from build123d import *

# Parameters (mm, degrees)
F1_DEPTH = 8
F2_R     = 3.99999
F3_R     = 1
F4_DEPTH = 60
F6_R     = 3.99999
F5_R     = 3.5
F7_DEPTH = 2
F8_R     = 0.75
F9_DEPTH = 12


# Not quite as in the source:
# - a fillet or chamfer is up to 0.001 mm smaller than in the source, because OpenCascade refuses the exact size


with BuildPart() as f1:
    # F0 (on Top) → F1 (new body)
    with BuildSketch(Plane.XY):
        Polygon((-9.9077894302, -1.920078908), (-9.9077894302, -12.520078908), (8.0922105698, -12.520078908), (8.0922105698, -0.520078908), (28.0922105698, -0.520078908), (28.0922105698, 10.079921092), (14.0922105698, 10.079921092), (14.0922105698, 22.579921092), (28.0922105698, 22.579921092), (28.0922105698, 33.179921092), (-9.9077894302, 33.179921092), (-9.9077894302, 22.579921092), (0.0922105698, 22.579921092), (0.0922105698, -1.920078908), align=None)
    extrude(amount=F1_DEPTH)

    # F2 (radius 4 in the source; OpenCascade refuses exactly that, so slightly less here)
    f2_edges = [f1.edges().sort_by_distance(p)[0] for p in [
        (-9.907789, -7.220079, 8),
        (-9.907789, -7.220079, 0),
        (8.092211, -6.520079, 8),
        (8.092211, -6.520079, 0),
        (28.092211, 4.779921, 8),
        (28.092211, 4.779921, 0),
        (28.092211, 27.879921, 8),
        (28.092211, 27.879921, 0),
        (-9.907789, 27.879921, 8),
        (-9.907789, 27.879921, 0),
    ]]
    fillet(f2_edges, radius=F2_R)

    # F3 (on face) → F4 (cut)
    with BuildSketch(Plane(origin=(0, 33.179921092, 0), x_dir=(-1, 0, 0), z_dir=(0, 1, 0))):
        with Locations((-24.0922105698, 4)):
            Circle(F3_R)
        with Locations((5.9077894302, 4)):
            Circle(F3_R)
    extrude(amount=-F4_DEPTH, mode=Mode.SUBTRACT)

    # F6 (radius 4 in the source; OpenCascade refuses exactly that, so slightly less here)
    f6_edges = [f1.edges().sort_by_distance(p)[0] for p in [
        (0.092211, 10.329921, 8),
        (0.092211, 10.329921, 0),
        (14.092211, 16.329921, 8),
        (14.092211, 16.329921, 0),
    ]]
    fillet(f6_edges, radius=F6_R)

    # F5 (on face) → F7 (join)
    with BuildSketch(Plane.XZ.offset(0.520078908)):
        with Locations((17.0922105698, 4)):
            Circle(F5_R)
    extrude(amount=F7_DEPTH)

    # F8 (on face) → F9 (cut)
    with BuildSketch(Plane.XZ.offset(2.520078908)):
        with Locations((17.0922105698, 4)):
            Circle(F8_R)
    extrude(amount=-F9_DEPTH, mode=Mode.SUBTRACT)


solid = f1.part
Work out the finished part from the listing and answer in its coordinate system (mm). A direction names the side the tool comes from. Coordinates: 2 decimals unless noted, no trailing zeros. Write each loop counter-clockwise with the first axis right and the second up, starting at its lowest first coordinate (ties: lowest second). Pieces come first, ordered by that corner, then holes. Notation, with made-up numbers: M 88,61 L 124,61 A29 cw 124,83 Z; hole C -13.5,80 d3. An arc over 180 degrees is marked long. Use one line per item in the form item = value. Start each with the question number.
1. The part is cut by section A-A (y = 30.5). Give the number of separate pieces and of enclosed holes in the cut face, plus the area to 3 significant figures.
2. Each of these flat-tipped pins is pushed along its axis until it touches: P1, Ø4, axis at y = 19.5, z = 5, coming from the -X side; P2, Ø1.2, axis at x = 17, z = 4, coming from the -Y side; P3, Ø4, axis at x = 14.5, z = 2.5, coming from the -Y side. Where does it stop, or does it pass through?
3. The mould has two halves that part along Y. Classify faces 4 (the face through (26.95, 4.85, 6.8)), 5 (the face through (1.295, 10.158, 1.141)), 6 (the face through (15.9, -0.52, 7.5)): released by +Y, released by -Y, zero draft, split by the parting line, or undercut.
4. A tool of negligible diameter and unlimited length cuts with its end or side. For faces 1 (the face through (12.89, 16.42, 6.86)), 2 (the face through (6.95, -6.44, 1.2)), 3 (the face through (1.295, 10.158, 6.859)), from which of +Z, -Z, +X, -X, +Y, -Y can it reach the whole face along a straight path? Write none if from no direction.
5. Straight lines are drawn through the part: probe 1 along Y at (x, z) = (-3.5, 6); probe 2 along Y at (x, z) = (14, 7.5); probe 3 along Y at (x, z) = (11.5, 5.75). For each, find the intervals that lie inside material, in ascending order. Write a range as from..to.
6. The part is cut by section B-B (z = 5.75). Give the vertices of the cut face in (x, y), plus the area to 3 significant figures.
Evaluation:
q1.separate_pieces = 1
q1.enclosed_holes = 2
q1.area = 284 mm^2
q2.P1 = 0.09
q2.P2 = 9.48
q2.P3 = -2.52
q3.face_4 = zero draft
q3.face_5 = undercut
q3.face_6 = released by -Y
q4.face_1 = +Z, +X
q4.face_2 = -Z, -Y
q4.face_3 = +Z, -X
q5.probe_1 = -12.52..-1.92, 22.58..33.18
q5.probe_2 = -0.52..10.08, 22.58..33.18
q5.probe_3 = -0.52..33.18
q6.outline = M -9.5,-12.52 L 7.69,-12.52 L 7.69,-0.52 L 14.06,-0.52 L 14.06,-2.52 L 20.12,-2.52 L 20.12,-0.52 L 27.69,-0.52 L 27.69,10.08 L 13.69,10.08 L 13.69,22.58 L 27.69,22.58 L 27.69,33.18 L -9.5,33.18 L -9.5,22.58 L 0.5,22.58 L 0.5,-1.92 L -9.5,-1.92 Z
q6.area = 1,050 mm^2
